from build123d import *

# Parameters (mm, degrees)
BOSS_EXTRUDE1_DEPTH = 40
SKETCH2_R           = 15.05
CUT_EXTRUDE1_DEPTH  = 40
FILLET1_R           = 15
SKETCH3_R           = 15.05
BOSS_EXTRUDE2_DEPTH = 40


with BuildPart() as part:
    # Sketch1 → Boss-Extrude1 (new body)
    with BuildSketch(Plane.XY):
        with BuildLine():
            Line((-23.162738789, 19.065348982), (-65.942835362, 30.52824131))
            Line((-65.942835362, 30.52824131), (-74.725635473, -2.249614938))
            Line((-74.725635473, -2.249614938), (-25.7643439, -15.368753476))
            ThreePointArc((-25.7643439, -15.368753476), (29.91474065, -2.260153064), (-23.162738789, 19.065348982))
        make_face()
    extrude(amount=BOSS_EXTRUDE1_DEPTH)

    # Sketch2 → Cut-Extrude1 (cut)
    with BuildSketch(Plane(origin=(-69.157563319, 18.530713242, 0), x_dir=(0, 0, 1), z_dir=(-0.9659258262890691, 0.2588190451025179, 0))):
        with Locations(Location((20, -4.546311876, 0), (0, 0, 270))):
            Circle(SKETCH2_R)
    extrude(amount=-CUT_EXTRUDE1_DEPTH, mode=Mode.SUBTRACT)

    # Fillet1
    fillet1_edges = [part.edges().sort_by_distance(p)[0] for p in [
        (-50.244989687, -8.809184207, 40),
        (-50.244989687, -8.809184207, 0),
        (-44.552787075, 24.796795146, 0),
        (-44.552787075, 24.796795146, 40),
    ]]
    fillet(fillet1_edges, radius=FILLET1_R)

    # Sketch3 → Boss-Extrude2 (add)
    with BuildSketch(Plane.XY.offset(40)):
        Circle(SKETCH3_R)
    extrude(amount=BOSS_EXTRUDE2_DEPTH)


solid = part.part
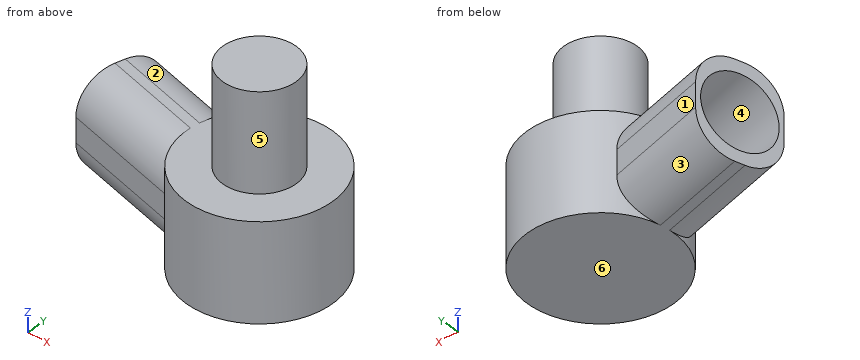
Geometry: final body of the model. Coordinates: model frame, mm. Face numbers are marked on the shaded views. A direction names the side the tool comes from. Give positions to 0.01 mm unless a question says otherwise; leave off trailing zeros. Write each loop counter-clockwise with the first axis right and the second up, starting at its lowest first coordinate (ties: lowest second). Pieces come first, ordered by that corner, then holes. Notation, with made-up numbers: M 40.25,55 L 69.25,55 A9 cw 69.25,62 Z; hole C -8.5,-34 d4. An arc over 180 degrees is marked long. Answer in a Markdown table with one row per item. Add a question column.
(1) Ray query, line 1 (Z direction, x = -6, y = 22); line 2 (Z direction, x = -67, y = 10.5); line 3 (Z direction, x = -35.5, y = 13). Return the intervals inside material, ascending.
(2) Section C-C on y = -21. Return loops of the section in (x, z), and give its area (3 significant figures).
(3) Section D-D on z = 63.5. Return loops of the section in (x, y).
(4) Section A-A on x = 0. Return loops of the section in (y, z).
(5) First-contact query: pin 1 (2 mm diameter, centred on x = -9.5, z = 56.5, fed in from +Y); pin 2 (4 mm diameter, centred on x = -11, z = 9.5, fed in from -Y); pin 3 (4 mm diameter, centred on x = -8.5, z = 15, fed in from +Y). Flat tips, straight axial feed; report the tip coordinate or a pass-through.
(6) Section B-B on z = 32. Return loops of the section in (x, y), and give its area (3 significant figures).
(7) Reachability of the marked faces 1, 2 and 3 from +Z, -Z, +X, -X, +Y, -Y: full face, straight path, thin tool, end or side. Return the list, or none.
(8) Mould query, pull axis Z, two halves, no side actions, for the marked faces 4, 5 and 6. Classes: +Z half, -Z half, draft (parallel to the pull), parting line (faces both ways), or undercut.
Result set:
| question | item | result |
|---|---|---|
| 1 | line 1 | z = 0 to 40 |
| 1 | line 2 | z = 0.02 to 5.19, 34.81 to 39.98 |
| 1 | line 3 | z = 1.23 to 7.2, 32.8 to 38.77 |
| 2 | outline | M -21.42,0 L 21.42,0 L 21.42,40 L -21.42,40 Z |
| 2 | area | 1,710 mm^2 |
| 3 | outline | C 0,0 d30.1 |
| 4 | outline | M -30,0 L 30,0 L 30,40 L 15.05,40 L 15.05,80 L -15.05,80 L -15.05,40 L -30,40 Z |
| 5 | pin 1 | stops at y = 12.42 |
| 5 | pin 2 | stops at y = -28.62 |
| 5 | pin 3 | stops at y = 29.29 |
| 6 | outline | M -74.28,-0.58 L -26.91,-13.27 A30 ccw long -24.31,17.58 L -66.39,28.85 L -67.98,22.91 L -29.35,12.56 L -34.05,-4.99 L -72.69,5.37 Z |
| 6 | area | 3,420 mm^2 |
| 7 | face 1 | +Z, -Z, +Y |
| 7 | face 2 | +Z, +Y |
| 7 | face 3 | -Z, +Y |
| 8 | face 4 | undercut |
| 8 | face 5 | draft |
| 8 | face 6 | -Z half |
